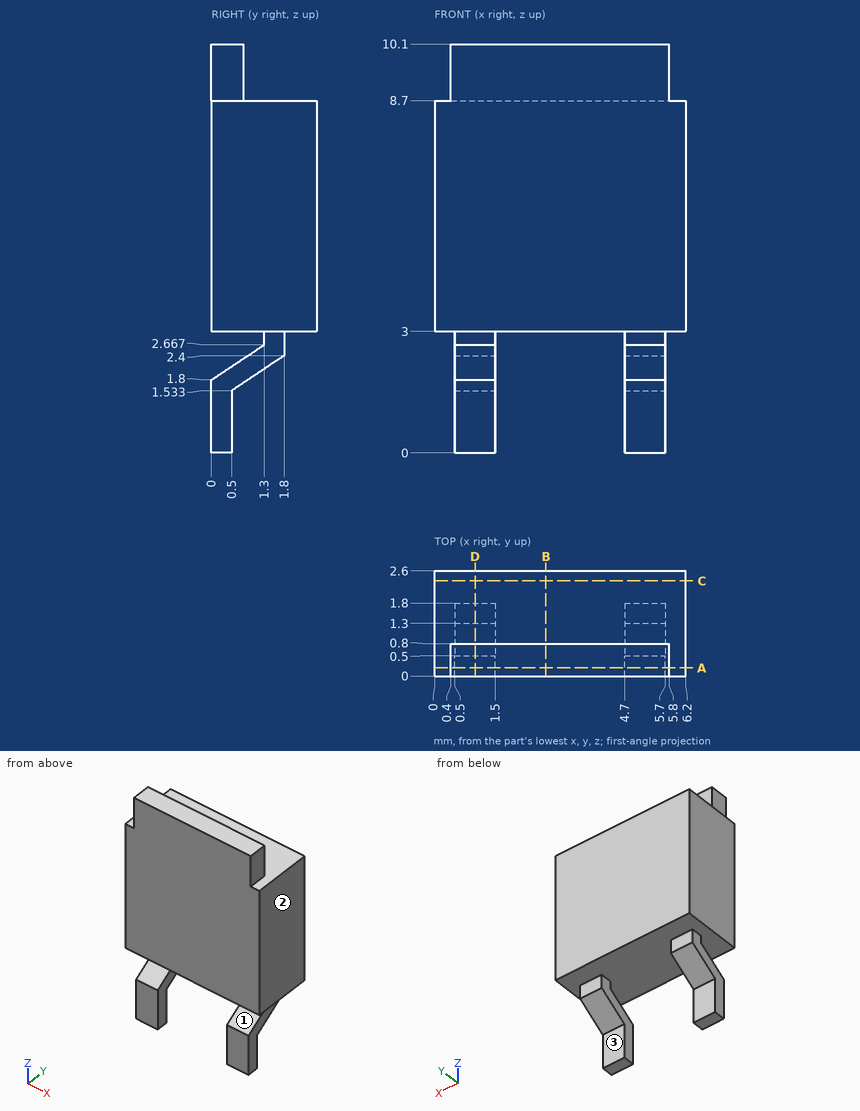
Source: three-view drawing plus pictorial views. Frame: mm from the lowest corner of the part. A direction names the side the tool comes from. Give positions to 0.01 mm unless a question says otherwise; leave off trailing zeros. Write each loop counter-clockwise with the first axis right and the second up, starting at its lowest first coordinate (ties: lowest second). Pieces come first, ordered by that corner, then holes.
(1) Ray query, line 1 (Z direction, x = 3, y = 0.9); line 2 (Y direction, x = 2.75, z = 9.25); line 3 (Z direction, x = 0.75, y = 0.4) (1 decimal). Return the intervals inside material, ascending.
(2) First-contact query: P1, Ø1.4, axis at y = 1, z = 2, coming from the -X side; P2, Ø0.6, axis at y = 0, z = 9.5, coming from the -X side; P3, Ø0.5, axis at y = 1.5, z = 2, coming from the +X side. Flat tips, straight axial feed; report the tip coordinate or a pass-through.
(3) Cut plane D-D, the plane x = 1. Return loops of the section in (y, z), then the cut area to 3 significant figures.
(4) Cut plane B-B, the plane x = 2.75. Return loops of the section in (y, z).
(5) Cut plane A-A, the plane y = 0.2. Return loops of the section in (x, z).
(6) Cut plane C-C, the plane y = 2.35. Return loops of the section in (x, z).
(7) Access query for the marked faces 1, 2 and 3. Directions: +Z, -Z, +X, -X, +Y, -Y. A direction counts if a zero-diameter tool reaches every point of the face in a straight line with its end or side. Return the directions, or none.
Values follow:
1. line 1: z = 3 to 8.7
1. line 2: y = 0 to 0.8
1. line 3: z = 0 to 2.1, 3 to 10.1
2. P1: stops at x = 0.5
2. P2: stops at x = 0.4
2. P3: stops at x = 5.7
3. outline: (0, 0) - (0.5, 0) - (0.5, 1.53) - (1.8, 2.4) - (1.8, 3) - (2.6, 3) - (2.6, 8.7) - (0.8, 8.7) - (0.8, 10.1) - (0, 10.1) - (0, 3) - (1.3, 3) - (1.3, 2.67) - (0, 1.8) - close
3. area: 17.8 mm2
4. outline: (0, 3) - (2.6, 3) - (2.6, 8.7) - (0.8, 8.7) - (0.8, 10.1) - (0, 10.1) - close
5. outline: (0, 3) - (6.2, 3) - (6.2, 8.7) - (5.8, 8.7) - (5.8, 10.1) - (0.4, 10.1) - (0.4, 8.7) - (0, 8.7) - close; (0.5, 0) - (1.5, 0) - (1.5, 1.93) - (0.5, 1.93) - close; (4.7, 0) - (5.7, 0) - (5.7, 1.93) - (4.7, 1.93) - close
6. outline: (0, 3) - (6.2, 3) - (6.2, 8.7) - (0, 8.7) - close
7. face 1: +X, -X, -Y
7. face 2: +Z, -Z, +X, +Y, -Y
7. face 3: -Z, +X, -X, +Y
